from build123d import *

# Parameters (mm, degrees)
BOSS_EXTRUDE1_DEPTH = 12
SKETCH2_R           = 5
BOSS_EXTRUDE2_DEPTH = 8
BOSS_EXTRUDE3_START = 8
SKETCH3_R           = 5
BOSS_EXTRUDE3_DEPTH = 8
SKETCH4_R           = 4
CUT_EXTRUDE1_DEPTH  = 30.415132160165456


with BuildPart() as part:
    # Sketch1 → Boss-Extrude1 (new body)
    with BuildSketch(Plane(origin=(0, 0, 0), x_dir=(1, 0, 0), z_dir=(0, 1, 0))):
        with BuildLine():
            Line((-4.330127018922256, 2.4999999999999996), (-7.499999999999998, 2.4999999999999996))
            Line((-7.499999999999998, 2.4999999999999996), (-7.499999999999998, -2.5000000000000004))
            Line((-7.499999999999998, -2.5000000000000004), (-4.330127018922255, -2.5000000000000004))
            ThreePointArc((-4.330127018922232, -2.4999999999999334), (-5, 6.1e-16), (-4.330127018922233, 2.4999999999999325))
        make_face()
        with BuildLine():
            ThreePointArc((4.330127018922173, 2.5000000000000346), (-5.965e-14, 5), (-4.330127018922233, 2.4999999999999325))
            Line((-4.330127018922256, 2.4999999999999996), (4.330127018922161, 2.4999999999999996))
        make_face()
        with BuildLine():
            Line((4.330127018922161, 2.4999999999999996), (-4.330127018922256, 2.4999999999999996))
            ThreePointArc((-4.330127018922233, 2.4999999999999325), (-5, 6.1e-16), (-4.330127018922232, -2.4999999999999334))
            Line((-4.330127018922255, -2.5000000000000004), (4.330127018922159, -2.5000000000000004))
            ThreePointArc((4.3301270189221714, -2.5000000000000364), (4.829629131445336, -1.294095225512625), (5, -1.22e-15))
            ThreePointArc((5, 0), (4.829629131445337, 1.2940952255126228), (4.330127018922173, 2.5000000000000346))
        make_face()
        with BuildLine():
            Line((7.500000000000002, 2.4999999999999996), (4.330127018922161, 2.4999999999999996))
            ThreePointArc((4.330127018922173, 2.5000000000000346), (4.829629131445337, 1.2940952255126228), (5, 0))
            ThreePointArc((5, -1.22e-15), (4.829629131445336, -1.294095225512625), (4.3301270189221714, -2.5000000000000364))
            Line((4.330127018922159, -2.5000000000000004), (7.500000000000002, -2.5000000000000004))
            Line((7.500000000000002, -2.5000000000000004), (7.500000000000002, 2.4999999999999996))
        make_face()
        with BuildLine():
            Line((4.330127018922159, -2.5000000000000004), (-4.330127018922255, -2.5000000000000004))
            ThreePointArc((-4.330127018922232, -2.4999999999999334), (-5.865e-14, -5), (4.3301270189221714, -2.5000000000000364))
        make_face()
    extrude(amount=BOSS_EXTRUDE1_DEPTH)

    # Sketch2 → Boss-Extrude2 (add)
    with BuildSketch(Plane(origin=(0, 12, 0), x_dir=(1, 0, 0), z_dir=(0, 1, 0))):
        with Locations(Location((0, 0, 0), (0, 0, 30))):
            Circle(SKETCH2_R)
    extrude(amount=BOSS_EXTRUDE2_DEPTH)

    # Sketch3 → Boss-Extrude3 (add)
    with BuildSketch(Plane.XZ.offset(BOSS_EXTRUDE3_START)):
        with Locations(Location((0, 0, 0), (0, 0, 270))):
            Circle(SKETCH3_R)
    extrude(amount=-BOSS_EXTRUDE3_DEPTH)

    # Sketch4 → Cut-Extrude1 (cut, through all)
    with BuildSketch(Plane.XZ.offset(8)):
        with Locations(Location((0, 0, 0), (0, 0, 270))):
            Circle(SKETCH4_R)
    extrude(amount=-CUT_EXTRUDE1_DEPTH, mode=Mode.SUBTRACT)


solid = part.part
Part model, mm, in its own coordinate system. A direction names the side the tool comes from. Give positions to 0.01 mm unless a question says otherwise; leave off trailing zeros. Order: outer loops, then holes, each group sorted by start corner. A loop starts at its lowest first (then second) coordinate and runs counter-clockwise, first axis right, second up. Notation, with made-up numbers: (23.25, -35) - (52.25, -35) arc R8 cw to (52.25, -20) - close; hole circle Ø2 at (19.5, 81.5). An arc over 180 degrees is marked (long way). Use a Markdown table: item, result.
1) Saw through at B-B on x = 0. List the corners of the cut face in (y, z).
Checked values:
| item | result |
|---|---|
| outline | (-8, -5) - (20, -5) - (20, -4) - (-8, -4) - close; (-8, 4) - (20, 4) - (20, 5) - (-8, 5) - close |
2) Saw through at D-D on x = -5.75. List the corners of the cut face in (y, z).
Checked values:
| item | result |
|---|---|
| outline | (0, -2.5) - (12, -2.5) - (12, 2.5) - (0, 2.5) - close |
3) 3-axis set-ups, long thin cutter, end or side, ignore diameter. For faces 1 (the flat face through (6, 6, 2.5)), 2 (the flat face through (-7.5, 6, 0)), 3 (the flat face through (-6, 6, -2.5)): which of +Z, -Z, +X, -X, +Y, -Y reach the whole face in a straight line?
Checked values:
| item | result |
|---|---|
| face 1 | +Z, +X, +Y, -Y |
| face 2 | +Z, -Z, -X, +Y, -Y |
| face 3 | -Z, -X, +Y, -Y |
4) Saw through at C-C on y = 5.5. List the corners of the cut face in (x, z), plus the area to 3 significant figures.
Checked values:
| item | result |
|---|---|
| outline | (-7.5, -2.5) - (-4.33, -2.5) arc R5 ccw to (4.33, -2.5) - (7.5, -2.5) - (7.5, 2.5) - (4.33, 2.5) arc R5 ccw to (-4.33, 2.5) - (-7.5, 2.5) - close; hole circle Ø8 at (0, 0) |
| area | 55.4 mm² |
5) Probe L1, parallel to X at y = 5.5, z = 0; L2, parallel to X at y = 14.25, z = 0; L3, parallel to Z at x = -5.5, y = 5.25. List the from-to ranges inside material, lowest first. Write a range as from..to.
Checked values:
| item | result |
|---|---|
| L1 | -7.5..-4, 4..7.5 |
| L2 | -5..-4, 4..5 |
| L3 | -2.5..2.5 |
6) Saw through at A-A on z = 0. List the corners of the cut face in (x, y), plus the area to 3 significant figures.
Checked values:
| item | result |
|---|---|
| outline | (-7.5, 0) - (-5, 0) - (-5, -8) - (-4, -8) - (-4, 20) - (-5, 20) - (-5, 12) - (-7.5, 12) - close; (4, -8) - (5, -8) - (5, 0) - (7.5, 0) - (7.5, 12) - (5, 12) - (5, 20) - (4, 20) - close |
| area | 116 mm² |
7) Two-plate mould, pull along Z, no slides. Class faces 4 (the flat face through (6, 6, -2.5)), 5 (the cylindrical face through (-3.905, 5.804, 0.867)), 6 (the flat face through (-4, 20, -2)), 7 (the flat face through (-6, 6, 2.5)): +Z half, -Z half, draft (parallel to the pull), parting line (faces both ways), or undercut.
Checked values:
| item | result |
|---|---|
| face 4 | -Z half |
| face 5 | undercut |
| face 6 | draft |
| face 7 | +Z half |
8) Flat gauge pins, fed straight in: P1, Ø1.5, axis at x = -5, z = -0.5, coming from the +Y side; P2, Ø6, axis at x = -3.5, y = 17, coming from the -Z side; P3, Ø2, axis at y = -5, z = 3.5, coming from the +X side; P4, Ø1.6, axis at x = 5.5, y = 3.5, coming from the -Z side. Where does each tip first touch, or does it go through?
Checked values:
| item | result |
|---|---|
| P1 | y = 20 |
| P2 | z = -4.97 |
| P3 | x = 4.33 |
| P4 | z = -2.5 |
